from build123d import *

# Parameters (mm, degrees)
F0_W     = 38.1
F0_H     = 19.05
F1_DEPTH = 3.175
F3_DEPTH = 3.176
F5_D     = 6.35


with BuildPart() as f1:
    # F0 (on Top) → F1 (new body)
    with BuildSketch(Plane.XY):
        with Locations((-19.05, 9.525)):
            Rectangle(F0_W, F0_H)
    extrude(amount=F1_DEPTH)

    # F2 (on face) → F3 (cut, through all)
    with BuildSketch(Plane.XY.offset(3.175)):
        with BuildLine():
            ThreePointArc((-38.1, 9.525), (-33.220058, 16.193908), (-25.465647, 19.05))
            Line((-25.465647, 19.05), (-38.1, 19.05))
            Line((-38.1, 19.05), (-38.1, 9.525))
        make_face()
        with BuildLine():
            ThreePointArc((-25.465647, 0), (-33.220058, 2.856092), (-38.1, 9.525))
            Line((-38.1, 9.525), (-38.1, 0))
            Line((-38.1, 0), (-25.465647, 0))
        make_face()
    extrude(amount=-F3_DEPTH, mode=Mode.SUBTRACT)

    # F5 (through all)
    with Locations(Plane.XY.offset(3.175)):
        with Locations((-32.890055, 10.653644)):
            Hole(F5_D / 2)


solid = f1.part
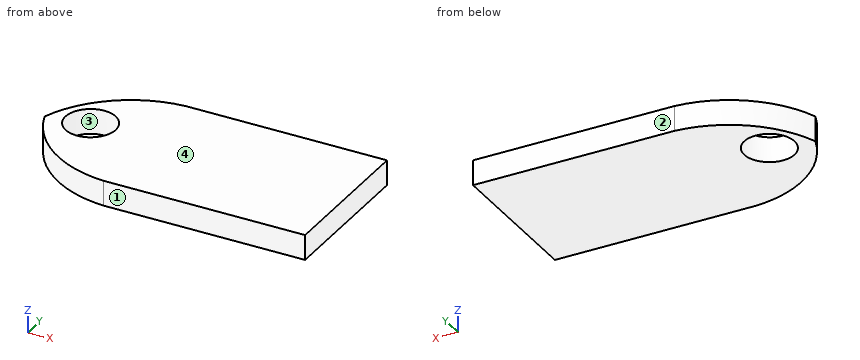
CAD build for the part. Positions are in the model's coordinates, mm. Face numbers are marked on the shaded views. Coordinates: 2 decimals unless noted, no trailing zeros. Order: outer loops, then holes, each group sorted by start corner. A loop starts at its lowest first (then second) coordinate and runs counter-clockwise, first axis right, second up.
Item 1: Band-saw the part on B-B on x = -31. List the corners of the cut face in (y, z) (1 decimal), plus the area to 3 significant figures.
Check sheet entries:
outline: (1.5, 0) - (8.1, 0) - (8.1, 3.2) - (1.5, 3.2) - close; (13.2, 0) - (17.6, 0) - (17.6, 3.2) - (13.2, 3.2) - close
area: 34.9 mm2
Item 2: Two-plate mould, pull along Y, no slides. Class the marked faces 1, 2, 3 and 4: +Y half, -Y half, draft (parallel to the pull), parting line (faces both ways), or undercut.
Check sheet entries:
face 1: -Y half
face 2: +Y half
face 3: undercut
face 4: draft
Item 3: Band-saw the part on A-A on y = 9. List the corners of the cut face in (x, z) (3 decimals).
Check sheet entries:
outline: (-37.903, 0) - (-35.6, 0) - (-35.6, 3.175) - (-37.903, 3.175) - close; (-30.18, 0) - (0, 0) - (0, 3.175) - (-30.18, 3.175) - close
Item 4: Band-saw the part on C-C on z = 1.95. List the corners of the cut face in (x, y) (3 decimals), plus the area to 3 significant figures.
Check sheet entries:
outline: (-38.1, 9.525) arc R14.301 ccw to (-25.466, 0) - (0, 0) - (0, 19.05) - (-25.466, 19.05) arc R14.301 ccw to start; hole circle Ø6.35 at (-32.89, 10.654)
area: 625 mm2
Item 5: Pin check, flat tip, straight feed: pin 1 Ø1.5 at (x, z) = (-31, 0.5) entering from -Y. Stop position of the tip, or through.
Check sheet entries:
pin 1: stops at y = 1.13
Item 6: Band-saw the part on D-D on y = 17. List the corners of the cut face in (x, z) (3 decimals), plus the area to 3 significant figures.
Check sheet entries:
outline: (-32.031, 0) - (0, 0) - (0, 3.175) - (-32.031, 3.175) - close
area: 102 mm2
Item 7: Drill centre lines: L1, parallel to X at y = 8, z = 0.3; L2, parallel to Y at x = -31, z = 1.3; L3, parallel to X at y = 11, z = 1.9. Where is each one in solid material? Low to high.
Check sheet entries:
L1: x = -37.46 to -34.63, -31.15 to 0
L2: y = 1.48 to 8.1, 13.2 to 17.57
L3: x = -37.49 to -36.05, -29.73 to 0
